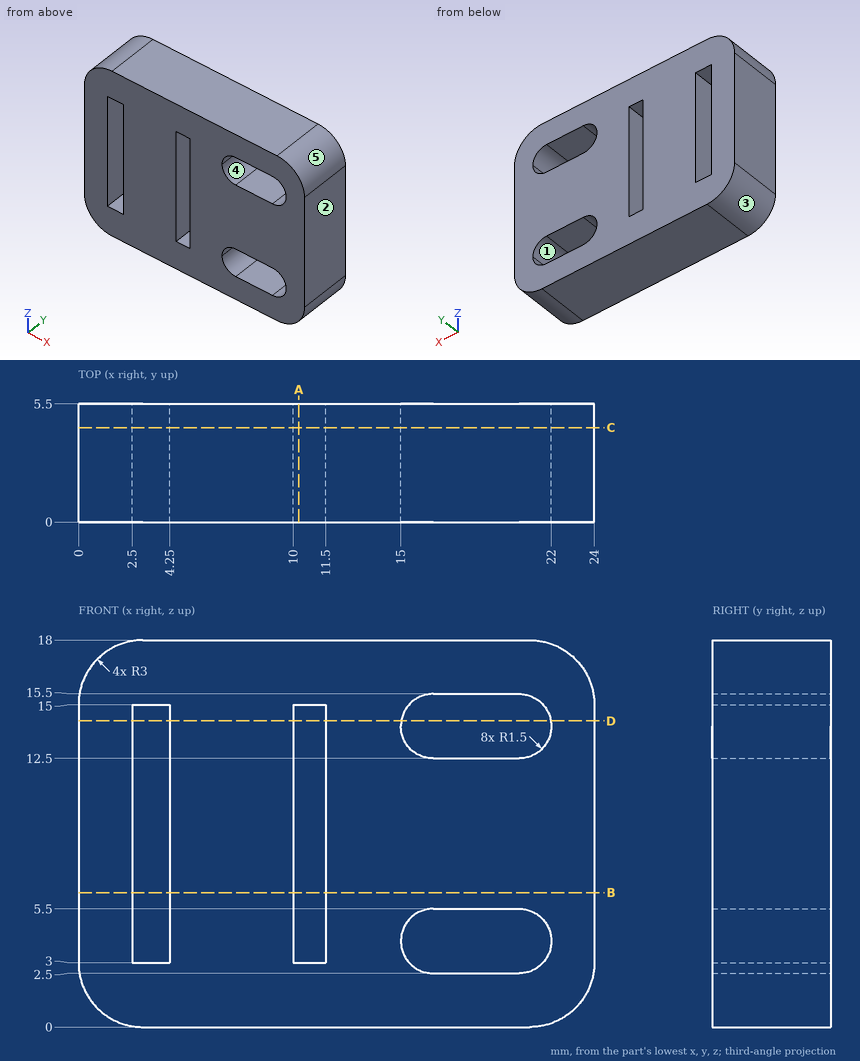
Geometry check sheet. Reference: drawing and pictorial views, mm from the part's lowest x, y, z. A direction names the side the tool comes from. Coordinates: 2 decimals unless noted, no trailing zeros. Write each loop counter-clockwise with the first axis right and the second up, starting at its lowest first coordinate (ties: lowest second). Pieces come first, ordered by that corner, then holes. Notation, with made-up numbers: (-23, -2) - (26, -2) arc R7 ccw to (26, 8) - close; hole circle Ø11 at (12.25, 31.25). An arc over 180 degrees is marked (long way). One line per question, with ' | ' between items. Start each with the question number.
1. Material ranges on line 1 along Z through (x, y) = (18.5, 3.95); line 2 along X through (y, z) = (4.85, 7); line 3 along Z through (x, y) = (11.25, 3.05), recorded low to high.
2. Section check C-C (y = 4.4). Count the separate pieces of the cut face and the enclosed holes in it, plus the area to 3 significant figures.
3. Draft check along X on the marked faces 1, 2 and 3. Enter one of: released by +X, released by -X, zero draft, split by the parting line, or undercut.
4. Section check B-B (z = 6.25). Enter the section's corners in (x, y).
5. Access from +Z, -Z, +X, -X, +Y, -Y to the whole of each face (thin tool, end or side, straight path). Record for the marked faces 4 and 5.
6. Section check A-A (x = 10.25). Enter the section's corners in (y, z).
7. Gauge pin test, flat end, axial feed: P1, Ø1, axis at x = 14.5, y = 2.5, coming from the -Z side. Record the tip position at first contact, or that the pin passes through.
8. Section check D-D (z = 14.25). Enter the section's corners in (x, y).
Computed values:
1) line 1: 0 to 2.5, 5.5 to 12.5, 15.5 to 18 | line 2: 0 to 2.5, 4.25 to 10, 11.5 to 24 | line 3: 0 to 3, 15 to 18
2) separate pieces: 1 | enclosed holes: 4 | area: 347 mm²
3) face 1: undercut | face 2: released by +X | face 3: released by -X
4) outline: (0, 0) - (2.5, 0) - (2.5, 5.5) - (0, 5.5) - close; (4.25, 0) - (10, 0) - (10, 5.5) - (4.25, 5.5) - close; (11.5, 0) - (24, 0) - (24, 5.5) - (11.5, 5.5) - close
5) face 4: +Y, -Y | face 5: +Z, +X, +Y, -Y
6) outline: (0, 0) - (5.5, 0) - (5.5, 3) - (0, 3) - close; (0, 15) - (5.5, 15) - (5.5, 18) - (0, 18) - close
7) P1: z = 0
8) outline: (0, 0) - (2.5, 0) - (2.5, 5.5) - (0, 5.5) - close; (4.25, 0) - (10, 0) - (10, 5.5) - (4.25, 5.5) - close; (11.5, 0) - (15.02, 0) - (15.02, 5.5) - (11.5, 5.5) - close; (21.98, 0) - (24, 0) - (24, 5.5) - (21.98, 5.5) - close
